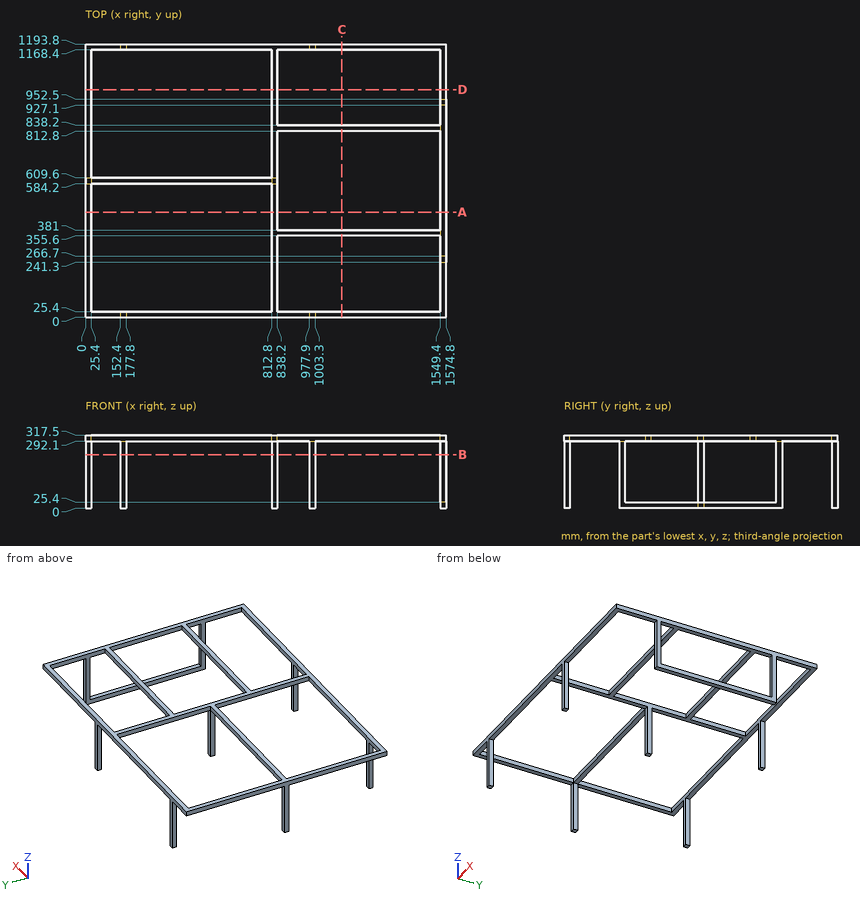
The figure shows three views and two pictorial views of one solid part (mm, origin at its lowest corner). Answer the questions. Coordinates: 2 decimals unless noted, no trailing zeros. Loops run counter-clockwise (first coordinate to the right, second up) from the corner with the lowest first, then second, coordinate; pieces in that order, holes last.
(1) The part is cut by section C-C (x = 1120). Determine the outline of the cut face in (y, z).
Solution:
outline: (0, 292.1) - (25.4, 292.1) - (25.4, 317.5) - (0, 317.5) - close; (355.6, 292.1) - (381, 292.1) - (381, 317.5) - (355.6, 317.5) - close; (812.8, 292.1) - (838.2, 292.1) - (838.2, 317.5) - (812.8, 317.5) - close; (1168.4, 292.1) - (1193.8, 292.1) - (1193.8, 317.5) - (1168.4, 317.5) - close
(2) The part is cut by section A-A (y = 460). Determine the outline of the cut face in (x, z).
Solution:
outline: (0, 292.1) - (25.4, 292.1) - (25.4, 317.5) - (0, 317.5) - close; (812.8, 292.1) - (838.2, 292.1) - (838.2, 317.5) - (812.8, 317.5) - close; (1549.4, 0) - (1574.8, 0) - (1574.8, 25.4) - (1549.4, 25.4) - close; (1549.4, 292.1) - (1574.8, 292.1) - (1574.8, 317.5) - (1549.4, 317.5) - close
(3) The part is cut by section B-B (z = 233.5). Count the separate pieces of the cut face and the enclosed holes in it, and give its area (3 significant figures).
Solution:
separate pieces: 8
enclosed holes: 0
area: 5,160 mm2
(4) Flat-ended cylindrical pins translate along their axes: pin 1 Ø2 at (x, y) = (836.5, 680) entering from -Z; pin 2 Ø12.5 at (y, z) = (1180, 104) entering from -X; pin 3 Ø7.5 at (x, z) = (1566.5, 173.5) entering from -Y; pin 4 Ø12 at (x, z) = (804.5, 38) entering from +Y. Find the tip coordinate at first contact, or state that the pin passes through.
Solution:
pin 1: stops at z = 292.1
pin 2: stops at x = 152.4
pin 3: stops at y = 241.3
pin 4: passes through
(5) The part is cut by section D-D (y = 994). Determine the outline of the cut face in (x, z).
Solution:
outline: (0, 292.1) - (25.4, 292.1) - (25.4, 317.5) - (0, 317.5) - close; (812.8, 292.1) - (838.2, 292.1) - (838.2, 317.5) - (812.8, 317.5) - close; (1549.4, 292.1) - (1574.8, 292.1) - (1574.8, 317.5) - (1549.4, 317.5) - close
(6) Consider line 1 along X through (y, z) = (626, 301.5); line 2 along Y through (x, z) = (996, 82.5); line 3 along Z through (x, y) = (948, 357.5). Determine where each line is inside the solid, lowest interval first.
Solution:
line 1: x = 0 to 25.4, 812.8 to 838.2, 1549.4 to 1574.8
line 2: y = 0 to 25.4, 1168.4 to 1193.8
line 3: z = 292.1 to 317.5
